The model under review builds one solid part; all positions refer to its coordinate system, in mm. Face numbers are marked on the shaded views. A direction names the side the tool comes from. Round coordinates to 2 decimals unless told otherwise and drop trailing zeros. Order: outer loops, then holes, each group sorted by start corner. A loop starts at its lowest first (then second) coordinate and runs counter-clockwise, first axis right, second up.
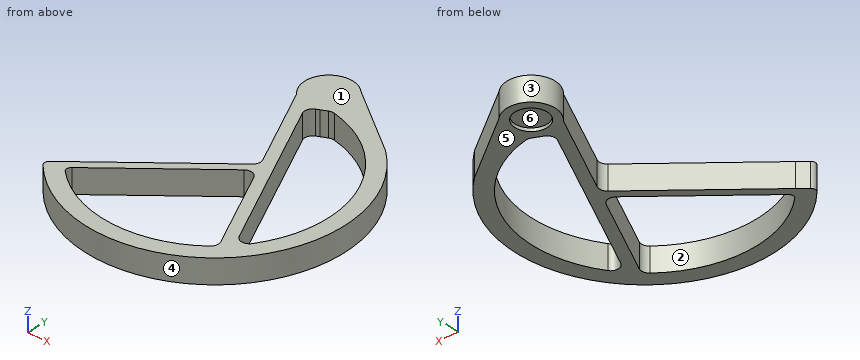
```python
from build123d import *

# Parameters (mm, degrees)
EXTRUDE_1_DEPTH     = 15
CUT_EXTRUDE_START   = -15
CUT_EXTRUDE_1_DEPTH = 15
SKETCH_8_R          = 10
CUT_EXTRUDE_3_DEPTH = 2


with BuildPart() as part:
    # Sketch 4 → Extrude 1 (new body)
    with BuildSketch(Plane.XY):
        with BuildLine():
            Line((-53.623111018, -124.995132678), (-58.940636287, -129.45706617))
            ThreePointArc((-58.940636287, -129.45706617), (-60.005384698, -131.552012131), (-59.233530865, -133.771635843))
            ThreePointArc((-59.233530865, -133.771635843), (57.362306223, -135.763481103), (52.076178918, -19.270504783))
            Line((52.076178918, -19.270504783), (10.606601718, 10.606601718))
            ThreePointArc((10.606601718, 10.606601718), (-10.606601718, 10.606601718), (-10.606601718, -10.606601718))
            Line((-10.606601718, -10.606601718), (14.536280154, -62.889638219))
            ThreePointArc((14.536280154, -62.889638219), (14.918089499, -66.109676181), (13.244185189, -68.886809092))
            Line((13.244185189, -68.886809092), (-53.623111018, -124.995132678))
        make_face()
        with BuildLine():
            Line((21.232400696, -76.813798404), (45.844843506, -127.993820346))
            ThreePointArc((45.844843506, -127.993820346), (46.221944165, -131.235480845), (44.518718993, -134.019289696))
            ThreePointArc((44.518718993, -134.019289696), (-2.231208213, -149.964431749), (-47.870174388, -131.072951785))
            ThreePointArc((-47.870174388, -131.072951785), (-48.817477846, -128.802229421), (-47.747678417, -126.586582094))
            Line((-47.747678417, -126.586582094), (13.511229465, -75.151532228))
            ThreePointArc((13.511229465, -75.151532228), (17.77869109, -74.092739753), (21.232400696, -76.813798404))
        make_face(mode=Mode.SUBTRACT)
    extrude(amount=EXTRUDE_1_DEPTH)

    # Sketch 6 → Cut-Extrude 1 (cut)
    with BuildSketch(Plane.XY.offset(15).offset(CUT_EXTRUDE_START)):
        with BuildLine():
            Line((49.189589797, -118.797265215), (2.201751786, -21.089020696))
            ThreePointArc((2.201751786, -21.089020696), (1.989274209, -17.268089629), (4.540836142, -14.416039025))
            Line((4.540836142, -14.416039025), (6.483415605, -13.48185369))
            Line((6.483415605, -13.48185369), (10.219658847, -11.685096486))
            ThreePointArc((10.219658847, -11.685096486), (11.747077013, -11.232198087), (13.339423466, -11.282754846))
            ThreePointArc((13.339423466, -11.282754846), (64.738421392, -53.37413296), (57.826055334, -119.448033215))
            ThreePointArc((57.826055334, -119.448033215), (53.319931874, -121.616182211), (49.189589797, -118.797265215))
        make_face()
    extrude(amount=CUT_EXTRUDE_1_DEPTH, mode=Mode.SUBTRACT)

    # Sketch 8 → Cut-Extrude 3 (cut)
    with BuildSketch(Plane(origin=(0, 0, 0), x_dir=(-1, 0, 0), z_dir=(0, 0, -1))):
        Circle(SKETCH_8_R)
    extrude(amount=-CUT_EXTRUDE_3_DEPTH, mode=Mode.SUBTRACT)


solid = part.part
```
(1) Insertion check: pin 1 (2 mm diameter, centred on y = -19.5, z = 13.5, fed in from +X); pin 2 (4 mm diameter, centred on x = -7.5, z = 9, fed in from +Y); pin 3 (6 mm diameter, centred on x = -5.5, z = 4.5, fed in from -Y). Each pin has a flat end and moves straight along its axis. Give the tip position at first contact, or say it passes through.
Data:
pin 1: stops at x = 53.48
pin 2: stops at y = 13.96
pin 3: stops at y = -159.96
(2) Consider section A-A (z = 6.5). Write out the cut boundary in (x, y), and give its area (3 significant figures).
Data:
outline: (-59.23, -133.77) arc R80 ccw (long way) to (52.08, -19.27) - (10.61, 10.61) arc R15 ccw to (-10.61, -10.61) - (14.54, -62.89) arc R5 cw to (13.24, -68.89) - (-58.94, -129.46) arc R3 ccw to start; hole (-47.87, -131.07) arc R70 ccw to (44.52, -134.02) arc R5 ccw to (45.84, -127.99) - (21.23, -76.81) arc R5 ccw to (13.51, -75.15) - (-47.75, -126.59) arc R3 ccw to start; hole (2.2, -21.09) - (49.19, -118.8) arc R5 ccw to (57.83, -119.45) arc R70 ccw to (13.34, -11.28) arc R5 ccw to (10.22, -11.69) - (4.54, -14.42) arc R5 ccw to start
area: 5,070 mm2
(3) Consider section C-C (y = -71.5). Write out the cut boundary in (x, z).
Data:
outline: (10.13, 0) - (26.44, 0) - (26.44, 15) - (10.13, 15) - close; (69.48, 0) - (79.55, 0) - (79.55, 15) - (69.48, 15) - close
(4) Consider section D-D (y = -96.5). Write out the cut boundary in (x, z), and give its area (3 significant figures).
Data:
outline: (-19.66, 0) - (-11.91, 0) - (-11.91, 15) - (-19.66, 15) - close; (30.7, 0) - (38.47, 0) - (38.47, 15) - (30.7, 15) - close; (68.03, 0) - (78.28, 0) - (78.28, 15) - (68.03, 15) - close
area: 387 mm2
(5) Consider section B-B (x = -33). Write out the cut boundary in (y, z).
Data:
outline: (-152.88, 0) - (-141.73, 0) - (-141.73, 15) - (-152.88, 15) - close; (-114.2, 0) - (-107.69, 0) - (-107.69, 15) - (-114.2, 15) - close
(6) For the marked faces 1 and 2, list the 3-axis set-ups (+Z, -Z, +X, -X, +Y, -Y) from which the entire face can be reached by the end or side of a thin tool; tool diameter is ignored.
Data:
face 1: +Z, +X, -X, +Y, -Y
face 2: +Z, -Z
(7) Draft analysis for pull direction Y (two halves, no side actions). For the marked faces 3, 4, 5 and 6, state which applies: pulls with the +Y half, pulls with the -Y half, needs draft (parallel to the pull), parting line crosses it, or undercut.
Data:
face 3: undercut
face 4: parting line crosses it
face 5: needs draft
face 6: undercut
(8) To check wall thickness, follow probe 1 along Y at (x, z) = (0, 1.6); probe 2 along Y at (x, z) = (16, 3.75); probe 3 along X at (y, z) = (-81, 7.75). State the ranges of each line that lie inside material, in increasing order.
Data:
probe 1: y = -160 to -150, -86.5 to -80, -32.66 to -10, 10 to 15
probe 2: y = -158.38 to -148.15, -74.03 to -49.78, -11.85 to 6.72
probe 3: x = -1.19 to 6.55, 23.25 to 31.01, 69.99 to 79.99
